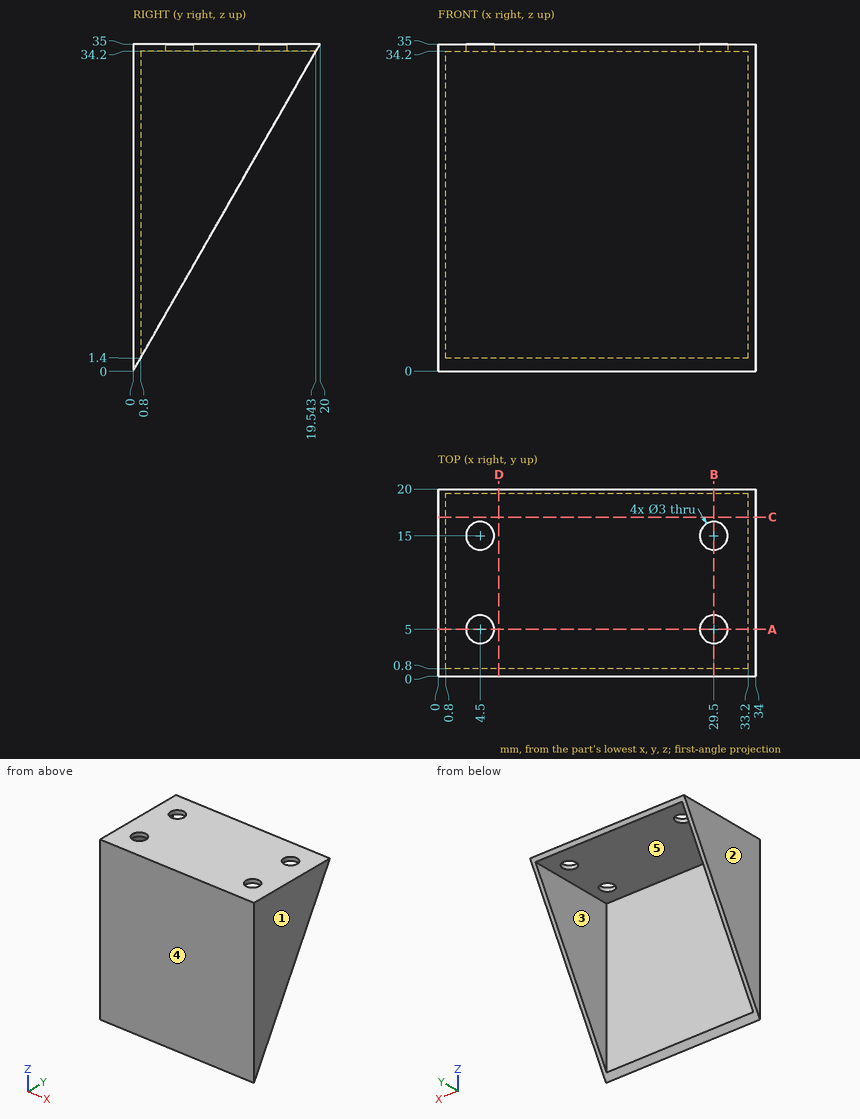
Drawing for the job (mm, zero at the part's lowest x, y, z). A direction names the side the tool comes from. Round coordinates to 2 decimals unless told otherwise and drop trailing zeros. Write each loop counter-clockwise with the first axis right and the second up, starting at its lowest first coordinate (ties: lowest second). Pieces come first, ordered by that corner, then holes. Notation, with made-up numbers: M -25.5,34.5 L 5.5,34.5 A9 cw 5.5,39.5 Z; hole C 28.25,86 d4. An arc over 180 degrees is marked long. Put each result on its own line as item: value.
Item 1: Cut at C-C (y = 17). List the corners of the cut face in (x, z).
Responses:
outline: M 0,29.75 L 0.8,29.75 L 0.8,34.2 L 33.2,34.2 L 33.2,29.75 L 34,29.75 L 34,35 L 0,35 Z
Item 2: Flat gauge pins, fed straight in: P1, Ø3.5, axis at x = 4.5, y = 15, coming from the -Z side; P2, Ø4, axis at x = 8, z = 20.5, coming from the +Y side; P3, Ø10, axis at x = 7, z = 28, coming from the -Y side; P4, Ø1.5, axis at y = 11.5, z = 15.5, coming from the +X side (3 decimals). Where does each tip first touch, or does it go through?
Responses:
P1: z = 34.2
P2: y = 0.8
P3: y = 0
P4: through
Item 3: Cut at A-A (y = 5). List the corners of the cut face in (x, z).
Responses:
outline: M 0,8.75 L 0.8,8.75 L 0.8,34.2 L 3,34.2 L 3,35 L 0,35 Z; M 6,34.2 L 28,34.2 L 28,35 L 6,35 Z; M 31,34.2 L 33.2,34.2 L 33.2,8.75 L 34,8.75 L 34,35 L 31,35 Z
Item 4: Cut at B-B (x = 29.5). List the corners of the cut face in (y, z).
Responses:
outline: M 0,0 L 0.8,1.4 L 0.8,34.2 L 3.5,34.2 L 3.5,35 L 0,35 Z; M 6.5,34.2 L 13.5,34.2 L 13.5,35 L 6.5,35 Z; M 16.5,34.2 L 19.54,34.2 L 20,35 L 16.5,35 Z
Item 5: Cut at D-D (x = 6.5). List the corners of the cut face in (y, z), and give its area (3 significant figures).
Responses:
outline: M 0,0 L 0.8,1.4 L 0.8,34.2 L 19.54,34.2 L 20,35 L 0,35 Z
area: 42.6 mm²
Item 6: Tool access for the marked faces 4 and 5: list every direction of +Z, -Z, +X, -X, +Y, -Y with a clear straight run to the whole face (end or side of a thin tool).
Responses:
face 4: +Z, -Z, +X, -X, -Y
face 5: -Z, +Y
Item 7: Probe L1, parallel to X at y = 5, z = 22; L2, parallel to Y at x = 29.5, z = 34.75; L3, parallel to Y at x = 32.5, z = 6.5. List the from-to ranges inside material, lowest first. Write a range as from..to.
Responses:
L1: 0..0.8, 33.2..34
L2: 0..3.5, 6.5..13.5, 16.5..19.86
L3: 0..0.8
Item 8: Mould opens along X. For the marked faces 1, 2 and 3 say: +X half, -X half, draft (parallel to the pull), parting line (faces both ways), or undercut.
Responses:
face 1: +X half
face 2: -X half
face 3: undercut
